from build123d import *

# Parameters (mm, degrees)
BOSS_EXTRUDE1_DEPTH = 50.8
SKETCH2_R           = 6.35
CUT_EXTRUDE1_DEPTH  = 85.29618662
FILLET1_R           = 2.54
CUT_EXTRUDE2_REACH  = 82.602
SKETCH3_R           = 6.35


with BuildPart() as part:
    # Sketch1 → Boss-Extrude1 (new body)
    with BuildSketch(Plane(origin=(0, 0, 0), x_dir=(0, 0, -1), z_dir=(1, 0, 0))):
        Polygon((12.7, 0), (14.2494, 0), (14.2494, 60.9346), (-14.2494, 60.9346), (-14.2494, 0), (-12.7, 0), (-12.7, 59.3852), (12.7, 59.3852), align=None)
    extrude(amount=BOSS_EXTRUDE1_DEPTH)

    # Sketch2 → Cut-Extrude1 (cut, through all)
    with BuildSketch(Plane.XY.offset(14.2494)):
        with Locations((9.525, 7.62)):
            Circle(SKETCH2_R)
        Polygon((22.86, 0), (50.8, 0), (50.8, 55.8546), (43.18, 55.8546), align=None)
    extrude(amount=-CUT_EXTRUDE1_DEPTH, mode=Mode.SUBTRACT)

    # Fillet1
    fillet1_edges = [part.edges().sort_by_distance(p)[0] for p in [
        (0, 0, -13.4747),
        (50.8, 55.8546, 13.4747),
        (50.8, 55.8546, -13.4747),
        (22.86, 0, -13.4747),
        (22.86, 0, 13.4747),
        (43.18, 55.8546, -13.4747),
        (43.18, 55.8546, 13.4747),
        (0, 0, 13.4747),
    ]]
    fillet(fillet1_edges, radius=FILLET1_R)

    # Sketch3 → Cut-Extrude2 (cut, up to next)
    with BuildSketch(Plane(origin=(0, 60.9346, 0), x_dir=(1, 0, 0), z_dir=(0, 1, 0)), mode=Mode.PRIVATE) as cut_extrude2_sk1:
        with Locations(Location((25.4, 0, 0), (0, 0, 270))):
            Circle(SKETCH3_R)
    cut_extrude2_tool1 = extrude(cut_extrude2_sk1.sketch, amount=-CUT_EXTRUDE2_REACH, mode=Mode.PRIVATE) & part.part
    add(cut_extrude2_tool1.solids().sort_by_distance((25.4, 60.9346, 0))[0], mode=Mode.SUBTRACT)


solid = part.part
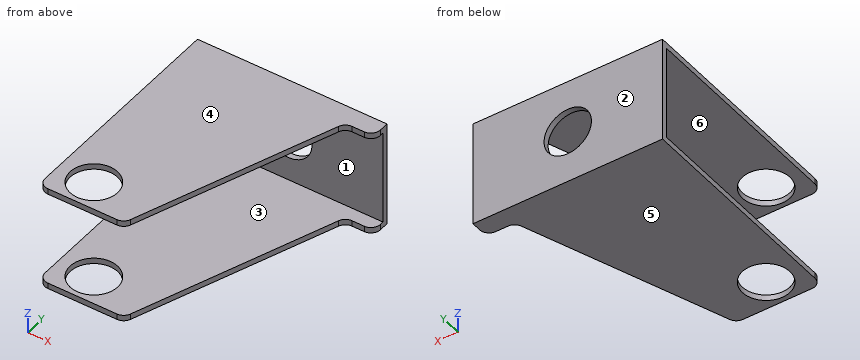
Read the model definition and answer for the solid it produces. Units are mm, in the model's axes. Face numbers are marked on the shaded views. A direction names the side the tool comes from. Coordinates: 2 decimals unless noted, no trailing zeros. Loops run counter-clockwise (first coordinate to the right, second up) from the corner with the lowest first, then second, coordinate; pieces in that order, holes last. Notation, with made-up numbers: (-13.5, 27) -> (13.5, 27) arc R24 cw to (13.5, 54) -> close; hole circle Ø7 at (14, 33). An arc over 180 degrees is marked (long way). Write item = value, one per line. Start each with the question number.
1) Find the intervals of material crossed by L1, parallel to Z at x = 9.5, y = 49; L2, parallel to Z at x = 25, y = 60; L3, parallel to Y at x = 41, z = 0.5, in increasing order. Write a range as from..to.
2) The part is cut by section C-C, the plane y = 33. Determine the outline of the cut face in (x, z), plus the area to 3 significant figures.
3) The part is cut by section B-B, the plane x = 25.4. Determine the outline of the cut face in (y, z).
4) For the marked faces 1 and 2, determine the directions among +Z, -Z, +X, -X, +Y, -Y from which every point of the face is accessible in a straight line to the end or side of a thin tool.
5) The mould has two halves that part along Z. Classify the marked faces 3, 4, 5 and 6: pulls with the +Z half, pulls with the -Z half, needs draft (parallel to the pull), parting line crosses it, or undercut.
6) Given P1, Ø1.2, axis at x = 47, z = -14, coming from the -Y side; P2, Ø14.5, axis at x = 25.4, z = 0, coming from the -Y side; P3, Ø11.5, axis at x = 9.525, y = 7.62, coming from the -Z side, each flat-ended and moving along its own axis, determine where each tip first touches the part or whether it passes through.
7) The part is cut by section D-D, the plane y = 7.62. Determine the outline of the cut face in (x, z) (3 decimals), plus the area to 3 significant figures.
8) The part is cut by section A-A, the plane z = 0. Determine the outline of the cut face in (x, y), plus the area to 3 significant figures.
Result:
q1.L1 = -14.25..-12.7, 12.7..14.25
q1.L2 = -14.25..-6.34, 6.34..14.25
q1.L3 = 59.39..60.93
q2.outline = (0, -14.25) -> (34.87, -14.25) -> (34.87, -12.7) -> (0, -12.7) -> close; (0, 12.7) -> (34.87, 12.7) -> (34.87, 14.25) -> (0, 14.25) -> close
q2.area = 108 mm²
q3.outline = (6.98, -14.25) -> (60.93, -14.25) -> (60.93, -6.35) -> (59.39, -6.35) -> (59.39, -12.7) -> (6.98, -12.7) -> close; (6.98, 12.7) -> (59.39, 12.7) -> (59.39, 6.35) -> (60.93, 6.35) -> (60.93, 14.25) -> (6.98, 14.25) -> close
q4.face_1 = +X, -X, -Y
q4.face_2 = +Z, -Z, +X, -X, +Y
q5.face_3 = undercut
q5.face_4 = pulls with the +Z half
q5.face_5 = pulls with the -Z half
q5.face_6 = undercut
q6.P1 = 55.85
q6.P2 = 59.39
q6.P3 = through
q7.outline = (0, -14.249) -> (3.175, -14.249) -> (3.175, -12.7) -> (0, -12.7) -> close; (0, 12.7) -> (3.175, 12.7) -> (3.175, 14.249) -> (0, 14.249) -> close; (15.875, -14.249) -> (25.632, -14.249) -> (25.632, -12.7) -> (15.875, -12.7) -> close; (15.875, 12.7) -> (25.632, 12.7) -> (25.632, 14.249) -> (15.875, 14.249) -> close
q7.area = 40.1 mm²
q8.outline = (0, 59.39) -> (19.05, 59.39) -> (19.05, 60.93) -> (0, 60.93) -> close; (31.75, 59.39) -> (50.8, 59.39) -> (50.8, 60.93) -> (31.75, 60.93) -> close
q8.area = 59.0 mm²
